from build123d import *

# Parameters (mm, degrees)
SKETCH1_W           = 38
SKETCH1_H           = 92
BOSS_EXTRUDE1_DEPTH = 10
SKETCH4_W           = 7
SKETCH4_H           = 7
CUT_EXTRUDE3_DEPTH  = 3
SKETCH7_R           = 3
CUT_EXTRUDE4_DEPTH  = 8
SKETCH8_R           = 3
CUT_EXTRUDE5_DEPTH  = 11
SKETCH9_R           = 3
CUT_EXTRUDE6_DEPTH  = 11


with BuildPart() as part:
    # Sketch1 → Boss-Extrude1 (new body)
    with BuildSketch(Plane(origin=(0, 0, 0), x_dir=(0, 0, -1), z_dir=(1, 0, 0))):
        with Locations((1.34375, -37.65625)):
            Rectangle(SKETCH1_W, SKETCH1_H)
    extrude(amount=BOSS_EXTRUDE1_DEPTH)

    # Sketch4 → Cut-Extrude3 (cut)
    with BuildSketch(Plane.ZY):
        with Locations((-1.34375, -4.15625)):
            Rectangle(SKETCH4_W, SKETCH4_H)
    extrude(amount=-CUT_EXTRUDE3_DEPTH, mode=Mode.SUBTRACT)

    # Sketch7 → Cut-Extrude4 (cut, through all)
    with BuildSketch(Plane.ZY.offset(-3)):
        with Locations((-1.34375, -4.15625)):
            Circle(SKETCH7_R)
    extrude(amount=-CUT_EXTRUDE4_DEPTH, mode=Mode.SUBTRACT)

    # Sketch8 → Cut-Extrude5 (cut, through all)
    with BuildSketch(Plane.ZY):
        with Locations((-1.34375, -76.15625)):
            Circle(SKETCH8_R)
    extrude(amount=-CUT_EXTRUDE5_DEPTH, mode=Mode.SUBTRACT)

    # Sketch9 → Cut-Extrude6 (cut, through all)
    with BuildSketch(Plane.ZY):
        with Locations((10.15625, -21.65625)):
            Circle(SKETCH9_R)
        with Locations((-12.84375, -21.65625)):
            Circle(SKETCH9_R)
    extrude(amount=-CUT_EXTRUDE6_DEPTH, mode=Mode.SUBTRACT)


solid = part.part
Source: CAD feature listing. Evaluate the final solid. Frame: model axes, mm. A direction names the side the tool comes from. Give positions to 0.01 mm unless a question says otherwise; leave off trailing zeros. Write each loop counter-clockwise with the first axis right and the second up, starting at its lowest first coordinate (ties: lowest second). Pieces come first, ordered by that corner, then holes. Notation, with made-up numbers: M 12.5,11.5 L 60.5,11.5 A35 ccw 60.5,47.5 Z; hole C -31.5,23 d6. An arc over 180 degrees is marked long. Answer as a JSON object with one key per item and string values.
Q1. Contact query for flat-ended pins moving along their axis: P1, Ø2, axis at y = -56, z = -5.5, coming from the -X side; P2, Ø5.5, axis at y = -4.5, z = -1, coming from the -X side. Output: stop coordinate, or through.
Geometry check:
{"P1": "stops at x = 0", "P2": "stops at x = 3"}
Q2. Cut plane C-C, the plane z = 9. Return the cut outline in (x, y), then the cut area to 3 significant figures.
Geometry check:
{"outline": "M 0,-83.66 L 10,-83.66 L 10,-24.42 L 0,-24.42 Z; M 0,-18.89 L 10,-18.89 L 10,8.34 L 0,8.34 Z", "area": "865 mm^2"}
Q3. Access query for faces 1 (the face through (3, -4.1, -4.5)), 2 (the face through (4.93, -23.482, -15.224)). Directions: +Z, -Z, +X, -X, +Y, -Y. A direction counts if a zero-diameter tool reaches every point of the face in a straight line with its end or side. Return the directions, or none.
Geometry check:
{"face 1": "-X", "face 2": "+X, -X"}
Q4. Cut plane A-A, the plane z = -15. Return the cut outline in (x, y).
Geometry check:
{"outline": "M 0,-83.66 L 10,-83.66 L 10,-23.74 L 0,-23.74 Z; M 0,-19.57 L 10,-19.57 L 10,8.34 L 0,8.34 Z"}
Q5. Ray query, line 1 along Y through (x, z) = (5, -1); line 2 along Y through (x, z) = (8.5, -0.5); line 3 along Y through (x, z) = (1.5, -12). Return the intervals inside material, ascending.
Geometry check:
{"line 1": "y = -83.66 to -79.14, -73.18 to -7.14, -1.18 to 8.34", "line 2": "y = -83.66 to -79.04, -73.28 to -7.04, -1.28 to 8.34", "line 3": "y = -83.66 to -24.54, -18.78 to 8.34"}
Q6. Mould query, pull axis Z, two halves, no side actions, for faces 3 (the face through (1, -7.656, -1)), 4 (the face through (5, -38, 17.656)), 5 (the face through (5, 8.344, -1)). Classes: +Z half, -Z half, draft (parallel to the pull), parting line (faces both ways), or undercut.
Geometry check:
{"face 3": "undercut", "face 4": "+Z half", "face 5": "draft"}
Q7. Cut plane B-B, the plane x = 5. Return the cut outline in (y, z), then the cut area to 3 significant figures.
Geometry check:
{"outline": "M -83.66,-20.34 L 8.34,-20.34 L 8.34,17.66 L -83.66,17.66 Z; hole C -76.16,-1.34 d6; hole C -21.66,-12.84 d6; hole C -21.66,10.16 d6; hole C -4.16,-1.34 d6", "area": "3,380 mm^2"}
